Work out the finished part from the listing and answer in its coordinate system (mm). A direction names the side the tool comes from. Coordinates: 2 decimals unless noted, no trailing zeros. Loops run counter-clockwise (first coordinate to the right, second up) from the corner with the lowest first, then second, coordinate; pieces in that order, holes last. Notation, with made-up numbers: (77, -36) - (132, -36) arc R27 ccw to (132, -10) - close; hole circle Ø11 at (-33.75, 23.25). An arc over 180 degrees is marked (long way). Write each question's results on one line, items separated by ' | '. Start each with the question number.
1. Determine the mould class of faces 1 (the flat face through (26.83, 14.92, -40.7)), 2 (the flat face through (16, 9, -82.55)), 3 (the cylindrical face through (-8.626, 0.258, -63.576)) for opening direction X: released by +X, released by -X, zero draft, split by the parting line, or undercut.
2. Which of the six approach directions +Z, -Z, +X, -X, +Y, -Y give full straight-line access (tool end or side, diameter ignored) to faces 4 (the flat face through (-8, 0, -42)), 5 (the flat face through (-8, 0.508, -42))?
3. Find the intervals of material crossed by line 1 along Y through (x, z) = (-1, -7.5); line 2 along X through (y, z) = (13.5, -52); line 3 along Y through (x, z) = (5.5, -48), in increasing order. Write a range as [from, to].
4. A cutting plane is placed at C-C on y = 9. Determine the outline of the cut face in (x, z).
5. A cutting plane is placed at B-B on x = -1.5. Determine the outline of the cut face in (y, z).
6. Each of these flat-tipped pins is pushed along its axis until it touches: P1, Ø4, axis at x = 41.5, z = -33.5, coming from the -Y side; P2, Ø5, axis at x = -7.94, z = -66.68, coming from the +Y side; P3, Ø4, axis at x = -8, z = -42, coming from the -Y side; P4, Ø12.5, axis at x = -9.5, z = -53.5, coming from the +Y side. Where does it stop, or does it pass through?
from build123d import *

# Parameters (mm, degrees)
SKETCH2_W                   = 15.875
SKETCH2_H                   = 82.55
BOSS_EXTRUDE2_DEPTH         = 0.508
EDGE_FLANGE2_DEPTH          = 82.55
F_1_4_0_25_DIAMETER_HOLE1_D = 6.35


# Sheet-metal steps are written as plain solids
with BuildPart() as part:
    # Sketch2 → Boss-Extrude2 (new body)
    with BuildSketch(Plane(origin=(0, 0, 0), x_dir=(1, 0, 0), z_dir=(0, 1, 0))):
        with Locations((-7.9375, 41.275)):
            Rectangle(SKETCH2_W, SKETCH2_H)
    extrude(amount=BOSS_EXTRUDE2_DEPTH)

    # Edge-Flange2 section (across the edge) → Edge-Flange2 (add)
    with BuildSketch(Plane(origin=(0.850738686, 0.508, 0), x_dir=(-0.49999999999999495, 0.8660254037844416, 0), z_dir=(0, 0, -1))):
        with BuildLine():
            Line((-0.508, 0.850738686), (-0.508, 59.380374))
            Line((-0.508, 59.380374), (0, 59.380374))
            Line((0, 59.380374), (0, 0.850738686))
            ThreePointArc((0, 0.850738686), (0.108185502, 0.028988218), (0.425369343, -0.736761314))
            Line((0.425369343, -0.736761314), (-0.014571562, -0.990761314))
            ThreePointArc((-0.014571562, -0.990761314), (-0.382504818, -0.102491857), (-0.508, 0.850738686))
        make_face()
    extrude(amount=EDGE_FLANGE2_DEPTH)

    # 1/4 (0.25) Diameter Hole1 (through all)
    with Locations(Plane(origin=(0, 0, 0), x_dir=(-1, 0, 0), z_dir=(0, -1, 0))):
        with Locations((7.9375, 15.875), (7.9375, 66.675)):
            Hole(F_1_4_0_25_DIAMETER_HOLE1_D / 2)


solid = part.part
Values:
1) face 1: released by +X | face 2: zero draft | face 3: undercut
2) face 4: +Z, -Z, +X, -X, -Y | face 5: +Z, -Z, -X, +Y
3) line 1: [0, 0.51] | line 2: [23.35, 24.37] | line 3: [2.61, 3.19]
4) outline: (15.56, -82.55) - (16.58, -82.55) - (16.58, 0) - (15.56, 0) - close
5) outline: (0, -82.55) - (0.51, -82.55) - (0.51, 0) - (0, 0) - close
6) P1: y = 22.24 | P2: through | P3: y = 0 | P4: y = 0.51
